```python
from build123d import *

# Parameters (mm, degrees)
F1_DEPTH = 0.5
F0_W     = 23
F0_H     = 12.5
F2_DEPTH = 5.5


with BuildPart() as f1:
    # F0 (on Top) → F1 (new body)
    with BuildSketch(Plane.XY):
        with BuildLine():
            Line((1.3369556665, 2.2427532598), (-18.6630443335, 2.2427532598))
            ThreePointArc((-18.6630443335, 2.2427532598), (-18.8094909429, 1.8891998692), (-19.1630443335, 1.7427532598))
            Line((-19.1630443335, 1.7427532598), (-19.1630443335, -7.7572467402))
            ThreePointArc((-19.1630443335, -7.7572467402), (-18.8094909429, -7.9036933496), (-18.6630443335, -8.2572467402))
            Line((-18.6630443335, -8.2572467402), (1.3369556665, -8.2572467402))
            ThreePointArc((1.3369556665, -8.2572467402), (1.4834022759, -7.9036933496), (1.8369556665, -7.7572467402))
            Line((1.8369556665, -7.7572467402), (1.8369556665, 1.7427532598))
            ThreePointArc((1.8369556665, 1.7427532598), (1.4834022759, 1.8891998692), (1.3369556665, 2.2427532598))
        make_face()
    extrude(amount=F1_DEPTH)

    # F0 (on Top) → F2 (join)
    with BuildSketch(Plane.XY):
        with Locations((-8.6630443335, -3.0072467402)):
            Rectangle(F0_W, F0_H)
        with BuildLine():
            ThreePointArc((-19.1630443335, 1.7427532598), (-19.5165977241, 2.5963066504), (-18.6630443335, 2.2427532598))
            Line((-18.6630443335, 2.2427532598), (1.3369556665, 2.2427532598))
            ThreePointArc((1.3369556665, 2.2427532598), (1.8369556665, 2.7427532598), (2.3369556665, 2.2427532598))
            ThreePointArc((2.3369556665, 2.2427532598), (2.1905090571, 1.8891998692), (1.8369556665, 1.7427532598))
            Line((1.8369556665, 1.7427532598), (1.8369556665, -7.7572467402))
            ThreePointArc((1.8369556665, -7.7572467402), (2.1905090571, -7.9036933496), (2.3369556665, -8.2572467402))
            ThreePointArc((2.3369556665, -8.2572467402), (1.8369556665, -8.7572467402), (1.3369556665, -8.2572467402))
            Line((1.3369556665, -8.2572467402), (-18.6630443335, -8.2572467402))
            ThreePointArc((-18.6630443335, -8.2572467402), (-19.5165977241, -8.6108001308), (-19.1630443335, -7.7572467402))
            Line((-19.1630443335, -7.7572467402), (-19.1630443335, 1.7427532598))
        make_face(mode=Mode.SUBTRACT)
    extrude(amount=F2_DEPTH)


solid = f1.part
```
Geometry check sheet. Reference: the model listing, model coordinates, mm. A direction names the side the tool comes from. Round coordinates to 2 decimals unless told otherwise and drop trailing zeros. Order: outer loops, then holes, each group sorted by start corner. A loop starts at its lowest first (then second) coordinate and runs counter-clockwise, first axis right, second up. Notation, with made-up numbers: (46.25, -34.75) - (77.25, -34.75) arc R5 ccw to (77.25, -25.75) - close; hole circle Ø5 at (-4.5, 25.25). An arc over 180 degrees is marked (long way). Use a Markdown table: item, result. Add a question column.
1) Section check A-A (z = 4.75). Record the cut outline in (x, y).
2) Thickness scan on line 1 along Y through (x, z) = (-17.5, 4.2); line 2 along X through (y, z) = (0.25, 5.2); line 3 along Z through (x, y) = (-9.5, 0). Record the ranges inside material, lowest first.
3) Mould release check, pull along X, two halves, no side actions. Record for faces 3 (the flat face through (-9, 3, 5.5)), 4 (the flat face through (1.837, -3, 3)), 5 (the flat face through (2.837, -3, 3)): released by +X, released by -X, zero draft, split by the parting line, or undercut.
4) Section check D-D (y = -4). Record the cut outline in (x, z), then the cut area to 3 significant figures.
5) Section check C-C (y = 2). Record the cut outline in (x, z).
6) Gauge pin test, flat ends, axial feed: P1, Ø1, axis at x = -12.5, y = -7, coming from the +Z side; P2, Ø0.9, axis at x = -19.16, y = 2.24, coming from the +Z side. Record the tip position at first contact, or that the pin passes through.
7) Section check B-B (x = -8.5). Record the cut outline in (y, z).
8) Set-up check for faces 1 (the flat face through (-9, -9.257, 3)), 2 (the flat face through (-9, -3, 0.5)): record each of +Z, -Z, +X, -X, +Y, -Y from which the full face is reachable in a straight line by a thin tool's end or side.
Established:
| question | item | result |
|---|---|---|
| 1 | outline | (-20.16, -9.26) - (2.84, -9.26) - (2.84, 3.24) - (-20.16, 3.24) - close; hole (-19.16, -7.76) arc R0.5 ccw (long way) to (-18.66, -8.26) - (1.34, -8.26) arc R0.5 ccw (long way) to (1.84, -7.76) - (1.84, 1.74) arc R0.5 ccw (long way) to (1.34, 2.24) - (-18.66, 2.24) arc R0.5 ccw (long way) to (-19.16, 1.74) - close |
| 2 | line 1 | -9.26 to -8.26, 2.24 to 3.24 |
| 2 | line 2 | -20.16 to -19.16, 1.84 to 2.84 |
| 2 | line 3 | 0 to 0.5 |
| 3 | face 3 | zero draft |
| 3 | face 4 | undercut |
| 3 | face 5 | released by +X |
| 4 | outline | (-20.16, 0) - (2.84, 0) - (2.84, 5.5) - (1.84, 5.5) - (1.84, 0.5) - (-19.16, 0.5) - (-19.16, 5.5) - (-20.16, 5.5) - close |
| 4 | area | 21.5 mm2 |
| 5 | outline | (-20.16, 0) - (-19.6, 0) - (-19.6, 5.5) - (-20.16, 5.5) - close; (-18.73, 0) - (1.4, 0) - (1.4, 0.5) - (-18.73, 0.5) - close; (2.27, 0) - (2.84, 0) - (2.84, 5.5) - (2.27, 5.5) - close |
| 6 | P1 | z = 0.5 |
| 6 | P2 | through |
| 7 | outline | (-9.26, 0) - (3.24, 0) - (3.24, 5.5) - (2.24, 5.5) - (2.24, 0.5) - (-8.26, 0.5) - (-8.26, 5.5) - (-9.26, 5.5) - close |
| 8 | face 1 | +Z, -Z, +X, -X, -Y |
| 8 | face 2 | +Z |
